from build123d import *

# Parameters (mm, degrees)
SKETCH_W              = 60
SKETCH_H              = 60
PAD_DEPTH             = 5
SKETCH001_R           = 2.25
PAD001_DEPTH          = 5
POLARPATTERN_COUNT    = 4
SKETCH002_W           = 10
SKETCH002_H           = 10
PAD002_DEPTH          = 100
POLARPATTERN001_COUNT = 4
SKETCH003_W           = 60
SKETCH003_H           = 60
PAD003_DEPTH          = 10


with BuildPart() as part:
    # Sketch → Pad (new body)
    with BuildSketch(Plane.XY):
        Rectangle(SKETCH_W, SKETCH_H)
    extrude(amount=PAD_DEPTH)

    # Sketch001 → Pad001 (join)
    with BuildSketch(Plane.XY):
        with Locations((-25, 25)):
            Circle(SKETCH001_R)
    pad001 = extrude(amount=-PAD001_DEPTH)

    # PolarPattern: Pad001 ×4 about axis
    polarpattern_axis = Axis((0, 0, 0), (0, 0, 1))
    for i in range(1, POLARPATTERN_COUNT):
        add(pad001.rotate(polarpattern_axis, i * 360 / POLARPATTERN_COUNT))

    # Sketch002 → Pad002 (join)
    with BuildSketch(Plane.XY):
        with Locations((25, 25)):
            Rectangle(SKETCH002_W, SKETCH002_H)
    pad002 = extrude(amount=PAD002_DEPTH)

    # PolarPattern001: Pad002 ×4 about axis
    polarpattern001_axis = Axis((0, 0, 0), (0, 0, 1))
    for i in range(1, POLARPATTERN001_COUNT):
        add(pad002.rotate(polarpattern001_axis, i * 360 / POLARPATTERN001_COUNT))

    # Sketch003 → Pad003 (join)
    with BuildSketch(Plane.XY.offset(100)):
        Rectangle(SKETCH003_W, SKETCH003_H)
    extrude(amount=PAD003_DEPTH)


solid = part.part
For this review, take the finished solid that the model builds, in its own axes (mm). A direction names the side the tool comes from. Round coordinates to 2 decimals unless told otherwise and drop trailing zeros. Loops run counter-clockwise (first coordinate to the right, second up) from the corner with the lowest first, then second, coordinate; pieces in that order, holes last. Notation, with made-up numbers: (19, 51) - (47, 51) arc R18 cw to (47, 77) - close; hole circle Ø9 at (80, -12.5). An arc over 180 degrees is marked (long way). Use one line per item in the form item = value.
Item 1: Consider section C-C on y = 5. Write out the cut boundary in (x, z).
Answers:
outline = (-30, 0) - (30, 0) - (30, 5) - (-30, 5) - close; (-30, 100) - (30, 100) - (30, 110) - (-30, 110) - close
Item 2: Mouldability with a two-part tool opening along Z and no side actions: class faces 1 (the flat face through (-20, 25, 52)), 2 (the flat face through (-20, -25, 52)), 3 (the flat face through (25, -25, -5)), 4 (the cylindrical face through (-23.962, 23.004, -2.465)) as +Z half, -Z half, draft (parallel to the pull), parting line (faces both ways), or undercut.
Answers:
face_1 = undercut
face_2 = undercut
face_3 = -Z half
face_4 = draft
Item 3: Tool access review of faces 5 (the flat face through (0, 0, 0)), 6 (the flat face through (0, 0, 5)), 7 (the flat face through (25, -20, 52)), 8 (the flat face through (25, 25, -5)), 9 (the flat face through (-20.4, 30, 66.5)): name each direction out of +Z, -Z, +X, -X, +Y, -Y from which nothing blocks a thin tool from reaching the whole face with its end or side.
Answers:
face_5 = -Z
face_6 = none
face_7 = +X, -X
face_8 = -Z, +X, -X, +Y, -Y
face_9 = +Z, -Z, +X, -X, +Y
Item 4: Clearance check with flat-ended pins moving along their axes: P1, Ø10, axis at x = -5, y = 4, coming from the -Z side; P2, Ø10, axis at y = 13.5, z = 69.5, coming from the -X side. State where each tip first meets the part, or that it passes through.
Answers:
P1 = 0
P2 = through
Item 5: For line 1 (Z direction, x = 6, y = 1); line 2 (X direction, y = -24, z = 79.5), list the stretches that pass through material, from the lowest coordinate up.
Answers:
line_1 = 0 to 5, 100 to 110
line_2 = -30 to -20, 20 to 30
Item 6: Consider section A-A on y = -25. Write out the cut boundary in (x, z), then the cut area to 4 significant figures.
Answers:
outline = (-30, 0) - (-27.25, 0) - (-27.25, -5) - (-22.75, -5) - (-22.75, 0) - (22.75, 0) - (22.75, -5) - (27.25, -5) - (27.25, 0) - (30, 0) - (30, 110) - (-30, 110) - close; hole (-20, 5) - (20, 5) - (20, 100) - (-20, 100) - close
area = 2,845 mm^2
